from build123d import *

# Parameters (mm, degrees)
ESBO_O1_R                     = 2.5
RESSALTO_EXTRUS_O1_DEPTH      = 10.6
ESBO_O8_W                     = 21.2
ESBO_O8_H                     = 35
RESSALTO_EXTRUS_O6_DEPTH      = 1.5
RESSALTO_EXTRUS_O2_DEPTH      = 1.5
CORTE_EXTRUS_O1_DEPTH         = 48.855720661
CORTE_EXTRUS_O1_DEPTH_BACK    = 48.855720661
ESBO_O3_W                     = 15.2
ESBO_O3_H                     = 37.5
CORTE_EXTRUS_O2_DEPTH         = 48.855720661
CORTE_EXTRUS_O2_DEPTH_BACK    = 48.855720661
ESBO_O4_R                     = 0.85
ESBO_O5_W                     = 3
ESBO_O5_H                     = 5
RESSALTO_EXTRUS_O3_DEPTH      = 2.5
RESSALTO_EXTRUS_O4_DEPTH      = 2.5
RESSALTO_EXTRUS_O5_START      = -58.6
ESBO_O7_W                     = 20
ESBO_O7_H                     = 64
RESSALTO_EXTRUS_O5_DEPTH      = 3
NERVURA2_REACH                = 95.102
ESBO_O10_WALL_W               = 206.642418638
ESBO_O10_WALL_H               = 2
ESBO_O11_W                    = 18
ESBO_O11_H                    = 35
RESSALTO_EXTRUS_O7_DEPTH      = 3
ESBO_O12_W                    = 13
ESBO_O12_H                    = 23
CORTE_EXTRUS_O3_DEPTH         = 106.818334895
ESBO_O13_R                    = 0.85
CORTE_EXTRUS_O4_DEPTH         = 106.818334895
FILETE1_R                     = 2
RESSALTO_EXTRUS_O11_OUTLINE_W = 9.625094948
RESSALTO_EXTRUS_O11_OUTLINE_H = 16.625094948
RESSALTO_EXTRUS_O11_DEPTH     = 23.57
RESSALTO_EXTRUS_O11_TAPER     = 8
RESSALTO_EXTRUS_O9_START      = -28.42
ESBO_O19_W                    = 18
ESBO_O19_H                    = 35
RESSALTO_EXTRUS_O9_DEPTH      = 3
ESBO_O20_W                    = 13
ESBO_O20_H                    = 23
CORTE_EXTRUS_O6_DEPTH         = 3
ESBO_O21_R                    = 0.85
CORTE_EXTRUS_O7_DEPTH         = 3
FILETE2_R                     = 3
RESSALTO_EXTRUS_O10_OUTLINE_W = 6.070697746
RESSALTO_EXTRUS_O10_OUTLINE_H = 11.070697746
RESSALTO_EXTRUS_O10_DEPTH     = 5.73
RESSALTO_EXTRUS_O10_TAPER     = 15
RESSALTO_EXTRUS_O13_START     = -23.62
ESBO_O28_W                    = 18
ESBO_O28_H                    = 35
RESSALTO_EXTRUS_O13_DEPTH     = 3
ESBO_O29_W                    = 13
ESBO_O29_H                    = 23
CORTE_EXTRUS_O8_DEPTH         = 3
ESBO_O30_R                    = 0.85
CORTE_EXTRUS_O9_DEPTH         = 3
FILETE4_R                     = 3
RESSALTO_EXTRUS_O14_OUTLINE_W = 11.77096594
RESSALTO_EXTRUS_O14_OUTLINE_H = 17.77096594
RESSALTO_EXTRUS_O14_DEPTH     = 83.68
RESSALTO_EXTRUS_O14_DRAFT     = -3
ESBO_O25_W                    = 34.112547474
ESBO_O25_H                    = 27.312547474
RESSALTO_EXTRUS_O12_DEPTH     = 3
ESBO_O32_W                    = 44.955348873
ESBO_O32_H                    = 44.228030444
RESSALTO_EXTRUS_O15_DEPTH     = 3
FILETE3_R                     = 5


# Read off the part's stored shape, not the designer's step: Ressalto-extrus_o11, Ressalto-extrus_o10, Ressalto-extrus_o14
with BuildPart() as part:
    # Esbo_o1 → Ressalto-extrus_o1 (new, symmetric)
    with BuildSketch(Plane(origin=(0, 0, 0), x_dir=(0, 0, -1), z_dir=(1, 0, 0))):
        Circle(ESBO_O1_R)
    extrude(amount=RESSALTO_EXTRUS_O1_DEPTH, both=True)

    # Esbo_o8 → Ressalto-extrus_o6 (add, symmetric)
    with BuildSketch(Plane.XY):
        with Locations((0, -17.5)):
            Rectangle(ESBO_O8_W, ESBO_O8_H)
    extrude(amount=RESSALTO_EXTRUS_O6_DEPTH, both=True)

    # Esbo_o2 → Ressalto-extrus_o2 (add, symmetric)
    with BuildSketch(Plane.XY):
        with BuildLine():
            Line((-10.6, -36), (-10.6, -35))
            Line((-10.6, -35), (-7.6, -35))
            Line((-7.6, -35), (-7.6, -36))
            ThreePointArc((-7.6, -36), (0, -43.6), (7.6, -36))
            Line((7.6, -36), (7.6, -35))
            Line((7.6, -35), (10.6, -35))
            Line((10.6, -35), (10.6, -36))
            ThreePointArc((10.6, -36), (0, -46.6), (-10.6, -36))
        make_face()
    extrude(amount=RESSALTO_EXTRUS_O2_DEPTH, both=True)

    # Esbo_o3 → Corte-extrus_o1 (cut, two sides: drawn at the far end of the back side and taken through both)
    with BuildSketch(Plane.XY.offset(-CORTE_EXTRUS_O1_DEPTH_BACK)):
        with Locations((0, -16.25)):
            Rectangle(ESBO_O3_W, ESBO_O3_H)
    extrude(amount=CORTE_EXTRUS_O1_DEPTH + CORTE_EXTRUS_O1_DEPTH_BACK, mode=Mode.SUBTRACT)

    # Esbo_o4 → Corte-extrus_o2 (cut, two sides: drawn at the far end of the back side and taken through both)
    with BuildSketch(Plane(origin=(0, 0, 0), x_dir=(0, 0, -1), z_dir=(1, 0, 0)).offset(-CORTE_EXTRUS_O2_DEPTH_BACK)):
        Circle(ESBO_O4_R)
    extrude(amount=CORTE_EXTRUS_O2_DEPTH + CORTE_EXTRUS_O2_DEPTH_BACK, mode=Mode.SUBTRACT)

    # Esbo_o5 → Ressalto-extrus_o3 (add, symmetric)
    with BuildSketch(Plane(origin=(0, 0, 0), x_dir=(0, 0, -1), z_dir=(1, 0, 0))):
        with Locations((0, -47.6)):
            Rectangle(ESBO_O5_W, ESBO_O5_H)
    extrude(amount=RESSALTO_EXTRUS_O3_DEPTH, both=True)

    # Esbo_o6 → Ressalto-extrus_o4 (add, symmetric)
    with BuildSketch(Plane(origin=(0, 0, 0), x_dir=(0, 0, -1), z_dir=(1, 0, 0))):
        with BuildLine():
            ThreePointArc((-10, -61.6), (-1.868272016, -58.231727984), (1.5, -50.1))
            ThreePointArc((1.5, -50.1), (0, -48.6), (-1.5, -50.1))
            ThreePointArc((-1.5, -50.1), (-3.98959236, -56.11040764), (-10, -58.6))
            ThreePointArc((-10, -58.6), (-11.5, -60.1), (-10, -61.6))
        make_face()
    extrude(amount=RESSALTO_EXTRUS_O4_DEPTH, both=True)

    # Esbo_o7 → Ressalto-extrus_o5 (add)
    with BuildSketch(Plane(origin=(0, 0, 0), x_dir=(1, 0, 0), z_dir=(0, 1, 0)).offset(RESSALTO_EXTRUS_O5_START)):
        with Locations((0, -37)):
            Rectangle(ESBO_O7_W, ESBO_O7_H)
    extrude(amount=-RESSALTO_EXTRUS_O5_DEPTH)

    # Esbo_o10 wall → Nervura2 (add, up to next)
    with BuildSketch(Plane(origin=(0, -52.6, 8.5), x_dir=(0, -0.650791373456, 0.759256602365), z_dir=(0, -0.759256602365, -0.650791373456)), mode=Mode.PRIVATE) as nervura2_sk1:
        Rectangle(ESBO_O10_WALL_W, ESBO_O10_WALL_H)
    nervura2_tool1 = extrude(nervura2_sk1.sketch, amount=NERVURA2_REACH, mode=Mode.PRIVATE) - part.part
    add(nervura2_tool1.solids().sort_by_distance((0, -52.6, 8.5))[0])



with BuildPart() as body_2:
    # Esbo_o11 → Ressalto-extrus_o7 (new body)
    with BuildSketch(Plane(origin=(37.8, 0, 0), x_dir=(0, 0, -1), z_dir=(1, 0, 0))):
        with Locations((-55, -17.53)):
            Rectangle(ESBO_O11_W, ESBO_O11_H)
    extrude(amount=RESSALTO_EXTRUS_O7_DEPTH)

    # Esbo_o12 → Corte-extrus_o3 (cut, through all)
    with BuildSketch(Plane(origin=(40.8, 0, 0), x_dir=(0, 0, -1), z_dir=(1, 0, 0))):
        with Locations((-55, -17.53)):
            Rectangle(ESBO_O12_W, ESBO_O12_H)
    extrude(amount=-CORTE_EXTRUS_O3_DEPTH, mode=Mode.SUBTRACT)

    # Esbo_o13 → Corte-extrus_o4 (cut, through all)
    with BuildSketch(Plane(origin=(40.8, 0, 0), x_dir=(0, 0, -1), z_dir=(1, 0, 0))):
        with Locations((-55, -3.53)):
            Circle(ESBO_O13_R)
        with Locations((-55, -31.53)):
            Circle(ESBO_O13_R)
    extrude(amount=-CORTE_EXTRUS_O4_DEPTH, mode=Mode.SUBTRACT)

    # Filete1
    filete1_edges = [body_2.edges().sort_by_distance(p)[0] for p in [
        (39.3, -0.03, 64),
        (39.3, -0.03, 46),
        (39.3, -35.03, 46),
        (39.3, -35.03, 64),
    ]]
    fillet(filete1_edges, radius=FILETE1_R)

    # Ressalto-extrus_o11 outline → Ressalto-extrus_o11 (add)
    with BuildSketch(Plane(origin=(0, -58.6, 0), x_dir=(1, 0, 0), z_dir=(0, 1, 0))):
        with Locations((39.3, -55)):
            Rectangle(RESSALTO_EXTRUS_O11_OUTLINE_W, RESSALTO_EXTRUS_O11_OUTLINE_H)
    extrude(amount=RESSALTO_EXTRUS_O11_DEPTH, taper=RESSALTO_EXTRUS_O11_TAPER)


with BuildPart() as body_3:
    # Esbo_o19 → Ressalto-extrus_o9 (new body)
    with BuildSketch(Plane(origin=(0, 0, 0), x_dir=(0, 0, -1), z_dir=(1, 0, 0)).offset(RESSALTO_EXTRUS_O9_START)):
        with Locations((-53.9, -35.37)):
            Rectangle(ESBO_O19_W, ESBO_O19_H)
    extrude(amount=RESSALTO_EXTRUS_O9_DEPTH)

    # Esbo_o20 → Corte-extrus_o6 (cut)
    with BuildSketch(Plane.ZY.offset(28.42)):
        with Locations((53.9, -35.37)):
            Rectangle(ESBO_O20_W, ESBO_O20_H)
    extrude(amount=-CORTE_EXTRUS_O6_DEPTH, mode=Mode.SUBTRACT)

    # Esbo_o21 → Corte-extrus_o7 (cut)
    with BuildSketch(Plane.ZY.offset(28.42)):
        with Locations((53.9, -21.37)):
            Circle(ESBO_O21_R)
        with Locations((53.9, -49.37)):
            Circle(ESBO_O21_R)
    extrude(amount=-CORTE_EXTRUS_O7_DEPTH, mode=Mode.SUBTRACT)

    # Filete2
    filete2_edges = [body_3.edges().sort_by_distance(p)[0] for p in [
        (-26.92, -17.87, 62.9),
        (-26.92, -17.87, 44.9),
        (-26.92, -52.87, 44.9),
        (-26.92, -52.87, 62.9),
    ]]
    fillet(filete2_edges, radius=FILETE2_R)

    # Ressalto-extrus_o10 outline → Ressalto-extrus_o10 (add)
    with BuildSketch(Plane(origin=(0, -58.6, 0), x_dir=(1, 0, 0), z_dir=(0, 1, 0))):
        with Locations((-26.92, -53.9)):
            Rectangle(RESSALTO_EXTRUS_O10_OUTLINE_W, RESSALTO_EXTRUS_O10_OUTLINE_H)
    extrude(amount=RESSALTO_EXTRUS_O10_DEPTH, taper=RESSALTO_EXTRUS_O10_TAPER)


with BuildPart() as body_4:
    # Esbo_o28 → Ressalto-extrus_o13 (new body)
    with BuildSketch(Plane(origin=(0, 0, 0), x_dir=(0, 0, -1), z_dir=(1, 0, 0)).offset(RESSALTO_EXTRUS_O13_START)):
        with Locations((-72.03, 42.58)):
            Rectangle(ESBO_O28_W, ESBO_O28_H)
    extrude(amount=RESSALTO_EXTRUS_O13_DEPTH)

    # Esbo_o29 → Corte-extrus_o8 (cut)
    with BuildSketch(Plane(origin=(-20.62, 0, 0), x_dir=(0, 0, -1), z_dir=(1, 0, 0))):
        with Locations((-72.03, 42.58)):
            Rectangle(ESBO_O29_W, ESBO_O29_H)
    extrude(amount=-CORTE_EXTRUS_O8_DEPTH, mode=Mode.SUBTRACT)

    # Esbo_o30 → Corte-extrus_o9 (cut)
    with BuildSketch(Plane(origin=(-20.62, 0, 0), x_dir=(0, 0, -1), z_dir=(1, 0, 0))):
        with Locations((-72.03, 56.58)):
            Circle(ESBO_O30_R)
        with Locations((-72.03, 28.58)):
            Circle(ESBO_O30_R)
    extrude(amount=-CORTE_EXTRUS_O9_DEPTH, mode=Mode.SUBTRACT)

    # Filete4
    filete4_edges = [body_4.edges().sort_by_distance(p)[0] for p in [
        (-22.12, 60.08, 81.03),
        (-22.12, 60.08, 63.03),
        (-22.12, 25.08, 63.03),
        (-22.12, 25.08, 81.03),
    ]]
    fillet(filete4_edges, radius=FILETE4_R)


with BuildPart() as ressalto_extrus_o14_tool:
    # Ressalto-extrus_o14 outline → Ressalto-extrus_o14 (with draft: the straight prism first)
    with BuildSketch(Plane.XZ.offset(58.6)):
        with Locations((-22.12, 72.03)):
            Rectangle(RESSALTO_EXTRUS_O14_OUTLINE_W, RESSALTO_EXTRUS_O14_OUTLINE_H)
    extrude(amount=-RESSALTO_EXTRUS_O14_DEPTH)
    # Ressalto-extrus_o14: the draft: its side faces are tilted about the plane it starts from
    ressalto_extrus_o14_sides = [ressalto_extrus_o14_tool.faces().sort_by_distance(p)[0] for p in [
        (-22.12, -16.76, 80.91548297),
        (-28.00548297, -16.76, 72.03),
        (-22.12, -16.76, 63.14451703),
        (-16.23451703, -16.76, 72.03),
    ]]
    draft(ressalto_extrus_o14_sides, Plane.XZ.offset(58.6), RESSALTO_EXTRUS_O14_DRAFT)


with BuildPart() as body_4_1:
    add(body_4.part)

    # Ressalto-extrus_o14: add ressalto_extrus_o14_tool
    add(ressalto_extrus_o14_tool.part)


with BuildPart() as part_1:
    add(part.part)

    add(body_2.part)  # Ressalto-extrus_o12 merges body 2
    # Esbo_o25 → Ressalto-extrus_o12 (add)
    with BuildSketch(Plane(origin=(0, -58.6, 0), x_dir=(1, 0, 0), z_dir=(0, 1, 0))):
        with Locations((27.056273737, -55.343726263)):
            Rectangle(ESBO_O25_W, ESBO_O25_H)
    extrude(amount=-RESSALTO_EXTRUS_O12_DEPTH)


    add(body_3.part)  # Ressalto-extrus_o15 merges body 3

    add(body_4_1.part)  # Ressalto-extrus_o15 merges body 4
    # Esbo_o32 → Ressalto-extrus_o15 (add)
    with BuildSketch(Plane(origin=(0, -58.6, 0), x_dir=(1, 0, 0), z_dir=(0, 1, 0))):
        with Locations((-12.477674437, -63.801467748)):
            Rectangle(ESBO_O32_W, ESBO_O32_H)
    extrude(amount=-RESSALTO_EXTRUS_O15_DEPTH)

    # Filete3
    filete3_edges = [part_1.edges().sort_by_distance(p)[0] for p in [
        (-34.955348873, -60.1, 85.91548297),
        (-34.955348873, -60.1, 41.687452526),
        (10, -60.1, 85.91548297),
        (-10, -60.1, 41.687452526),
        (-10, -60.1, 5),
        (10, -60.1, 5),
        (10, -60.1, 69),
        (44.112547474, -60.1, 69),
        (10, -60.1, 41.687452526),
        (44.112547474, -60.1, 41.687452526),
    ]]
    fillet(filete3_edges, radius=FILETE3_R)


solid = part_1.part
Input: part model. Units: mm. Frame: model coordinates. A direction names the side the tool comes from. Coordinates: 2 decimals unless noted, no trailing zeros. Order: outer loops, then holes, each group sorted by start corner. A loop starts at its lowest first (then second) coordinate and runs counter-clockwise, first axis right, second up.
1. Cut plane B-B, the plane x = 26. Return loops of the section in (y, z).
Checked values:
outline: (-61.6, 41.69) - (-58.6, 41.69) - (-58.6, 69) - (-61.6, 69) - close
2. Cut plane C-C, the plane z = 7. Return loops of the section in (x, y).
Checked values:
outline: (-9, -61.6) - (9, -61.6) - (9, -58.6) - (2.5, -58.6) - (2.5, -58.05) - (1, -58.05) - (1, -51.31) - (-1, -51.31) - (-1, -58.05) - (-2.5, -58.05) - (-2.5, -58.6) - (-9, -58.6) - close
3. Draft query along Y for faces 5 (the flat face through (-22.2, -26.64, 79.24)), 6 (the flat face through (-5, -61.6, 54)), 7 (the flat face through (39, -6.03, 55)), 8 (the flat face through (-27, -36, 62.9)). Return one class per face: +Y half, -Y half, draft (parallel to the pull), parting line (faces both ways), or undercut.
Checked values:
face 5: undercut
face 6: -Y half
face 7: undercut
face 8: draft
4. Cut plane A-A, the plane z = 18. Return loops of the section in (x, y).
Checked values:
outline: (-10, -61.6) - (10, -61.6) - (10, -58.6) - (-10, -58.6) - close
5. Access query for faces 1 (the flat face through (-7.6, -16, 0)), 2 (the flat face through (1, -54, 7)), 3 (the flat face through (-22, 42, 63.03)), 4 (the flat face through (-27, -36, 47.4)). Directions: +Z, -Z, +X, -X, +Y, -Y. A direction counts if a zero-diameter tool reaches every point of the face in a straight line with its end or side. Return the directions, or none.
Checked values:
face 1: +Z, -Z, +Y
face 2: +Z, +X, +Y
face 3: -Z, +X, -X, +Y
face 4: -X
6. Contact query for flat-ended pins moving along their axis: P1, Ø1.5, axis at y = -19, z = 1, coming from the +X side; P2, Ø9, axis at y = 38, z = 71, coming from the -X side; P3, Ø9.5, axis at y = -55.5, z = 6.5, coming from the -X side; P4, Ø1.5, axis at x = -21.5, y = 38, coming from the -Z side. Output: stop coordinate, or through.
Checked values:
P1: stops at x = 10.6
P2: passes through
P3: stops at x = -10
P4: stops at z = 63.03
7. Ray query, line 1 along Y through (x, z) = (-22.1, 72.03); line 2 along Y through (x, z) = (38, 55); line 3 along Z through (x, y) = (9, 0). Return the intervals inside material, ascending.
Checked values:
line 1: y = -61.6 to 27.73, 29.43 to 31.08, 54.08 to 55.73, 57.43 to 60.08
line 2: y = -61.6 to -32.38, -30.68 to -29.03, -6.03 to -4.38, -2.68 to -0.03
line 3: z = -2.5 to -0.85, 0.85 to 2.5
